Autodesk Inventor part; units mm, degrees
ref_plane "Work Plane1" through (8, 0, 0) normal (1, 0, 0) x (0, 1, 0)
ref_plane "XZ Plane" through (0, 0, 0) normal (0, 1, 0) x (-1, 0, 0)
ref_plane "XY Plane" through (0, 0, 0) normal (0, 0, 1) x (1, 0, 0)
ref_plane "Work Plane1" through (8, 0, 0) normal (1, 0, 0) x (0, 1, 0)
sketch "Sketch4" plane through (8, 0, 0) normal (1, 0, 0) x (0, 1, 0)
  line L0 (-5, 0) -> (-5, 10)
  line L1 (15, 53) -> (15, -29)
  line L2 (-5, 0) -> (15, -2)
  line L3 (-5, 10) -> (15, 60)
  line L4 (15, 60) -> (15, -2)
  point P0 (0, 0)
  dimension "d9" = 10
  dimension "d10" = 20
  dimension "d11" = 2
  dimension "d12" = 60
sketch "Sketch5" plane through (0, 0, 0) normal (0, 1, 0) x (-1, 0, 0)
  line L0 (12.5, 65) -> (-12.5, 65)
  line L1 (-12.5, 65) -> (-12.5, -7)
  line L2 (-12.5, -7) -> (12.5, -7)
  line L3 (12.5, -7) -> (12.5, 65)
  line L4 (12.5, 65) -> (-12.5, -7) construction
  line L5 (-12.5, 65) -> (12.5, -7) construction
  point P0 (0, 0)
  point P1 (0, 29)
  dimension "d13" = 25
  dimension "d14" = 72
  dimension "d15" = 7
  dimension "d22" = 0
extrude "Extrusion2" add sketch "Sketch5" along normal blind 15 and the other way blind 10
extrude "Extrusion3" cut sketch "Sketch4" against normal blind 16
properties part number "Mould Design"
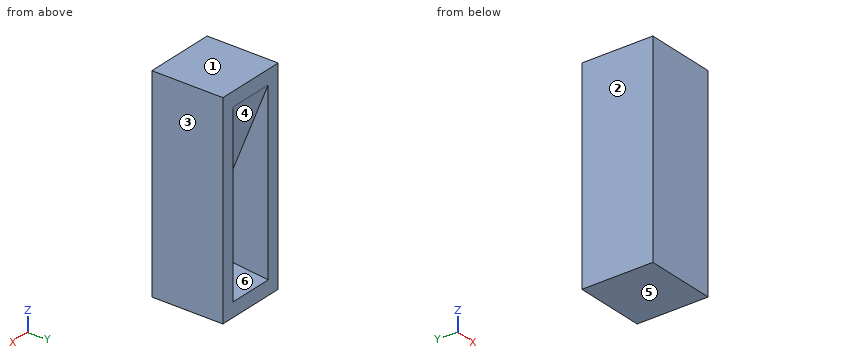
Here's how the part is built. I have some questions about the finished solid (model axes, mm). Face numbers are marked on the shaded views. A direction names the side the tool comes from. Coordinates: 2 decimals unless noted, no trailing zeros. Order: outer loops, then holes, each group sorted by start corner. A loop starts at its lowest first (then second) coordinate and runs counter-clockwise, first axis right, second up. Notation, with made-up numbers: (-20.5, -28.5) -> (-9.5, -28.5) arc R23 ccw to (-9.5, -8.5) -> close; hole circle Ø3 at (78.25, 73.25). An arc over 180 degrees is marked (long way). Answer in a Markdown table with one row per item.
(1) I want a section at C-C on x = 4.25. List the corners of the cut face in (y, z) for me.
Answer key:
| item | result |
|---|---|
| outline | (-10, -7) -> (15, -7) -> (15, -2) -> (-5, 0) -> (-5, 10) -> (15, 60) -> (15, 65) -> (-10, 65) -> close |
(2) Thinking about a two-plate mould opening in X: for the marked faces 1, 2, 3 and 4, which applies, +X half, -X half, draft (parallel to the pull), parting line (faces both ways), or undercut?
Answer key:
| item | result |
|---|---|
| face 1 | draft |
| face 2 | -X half |
| face 3 | +X half |
| face 4 | undercut |
(3) Will these pins go through, and if not, where does the flat tip stop? pin 1 Ø5 at (x, z) = (-0.5, 5.5) entering from +Y; pin 2 Ø10 at (x, z) = (-7.5, 26) entering from +Y.
Answer key:
| item | result |
|---|---|
| pin 1 | y = -5 |
| pin 2 | y = 15 |
(4) On a 3-axis mill with a long thin cutter (end or side, diameter ignored), from which of +Z, -Z, +X, -X, +Y, -Y can I reach the whole of each face in a straight line? I mean the marked faces 5 and 6. Say none if no direction works.
Answer key:
| item | result |
|---|---|
| face 5 | -Z, +X, -X, +Y, -Y |
| face 6 | +Y |
(5) I want a section at D-D on y = 11. List the corners of the cut face in (x, z) for me.
Answer key:
| item | result |
|---|---|
| outline | (-12.5, -7) -> (12.5, -7) -> (12.5, 65) -> (-12.5, 65) -> close; hole (-8, -1.6) -> (8, -1.6) -> (8, 50) -> (-8, 50) -> close |
(6) I want a section at A-A on y = 6.5. List the corners of the cut face in (x, z) for me, then the cut area to 3 significant figures.
Answer key:
| item | result |
|---|---|
| outline | (-12.5, -7) -> (12.5, -7) -> (12.5, 65) -> (-12.5, 65) -> close; hole (-8, -1.15) -> (8, -1.15) -> (8, 38.75) -> (-8, 38.75) -> close |
| area | 1,160 mm^2 |
(7) I want a section at B-B on z = 49.5. List the corners of the cut face in (x, y) for me.
Answer key:
| item | result |
|---|---|
| outline | (-12.5, -10) -> (12.5, -10) -> (12.5, 15) -> (8, 15) -> (8, 10.8) -> (-8, 10.8) -> (-8, 15) -> (-12.5, 15) -> close |
(8) Please list where these lines run through material, in increasing order: probe 1 along X at (y, z) = (10, 37); probe 2 along Y at (x, z) = (-4.5, 6); probe 3 along Y at (x, z) = (-6.5, 23.5).
Answer key:
| item | result |
|---|---|
| probe 1 | -12.5 to -8, 8 to 12.5 |
| probe 2 | -10 to -5 |
| probe 3 | -10 to 0.4 |
